from build123d import *

# Parameters (mm, degrees)
F0_W     = 20
F0_H     = 120
F1_DEPTH = 25
F2_R     = 2.5
F3_DEPTH = 20.001


with BuildPart() as f1:
    # F0 (on Front) → F1 (new body, symmetric)
    with BuildSketch(Plane.XZ):
        Rectangle(F0_W, F0_H)
        with BuildLine():
            ThreePointArc((87.128021, -54.795358), (51.166331, -95.96169), (10, -60))
            Line((10, -60), (-10, -60))
            ThreePointArc((-10, -60), (51.166331, -115.96169), (107.128021, -54.795358))
            Line((107.128021, -54.795358), (87.128021, -54.795358))
        make_face()
    extrude(amount=F1_DEPTH, both=True)

    # F2 (on face) → F3 (cut, through all)
    with BuildSketch(Plane.YZ.offset(10)):
        with Locations((0, -21.438537)):
            Circle(F2_R)
        with Locations((0, 38.03635)):
            Circle(F2_R)
    extrude(amount=-F3_DEPTH, mode=Mode.SUBTRACT)


solid = f1.part
Verification items for the finished model (mm, model axes). Coordinates: 2 decimals unless noted, no trailing zeros. Order: outer loops, then holes, each group sorted by start corner. A loop starts at its lowest first (then second) coordinate and runs counter-clockwise, first axis right, second up.
1. Release check for a two-part mould opening along X. For faces 1 (the face through (-10, 0, -1)), 2 (the face through (52.014, -0.35, -95.895)), 3 (the face through (50, 0, -116)), 4 (the face through (97, 0, -54.795)) record: +X half, -X half, draft (parallel to the pull), parting line (faces both ways), or undercut.
Results found:
face 1: -X half
face 2: undercut
face 3: parting line
face 4: draft
2. Go/stop test with flat-tipped pins: pin 1 Ø3 at (x, y) = (84, -17) entering from -Z; pin 2 Ø1 at (x, y) = (38.5, 9.5) entering from +Z; pin 3 Ø6 at (x, y) = (93.5, -0.5) entering from +Z. Record where each tip stops, or that it passes through.
Results found:
pin 1: stops at z = -105.2
pin 2: stops at z = -94.58
pin 3: stops at z = -54.8
3. Sectioned sample at D-D, the plane x = 39.5. Record the cut outline in (y, z).
Results found:
outline: (-25, -115.31) - (25, -115.31) - (25, -94.97) - (-25, -94.97) - close
4. Sectioned sample at B-B, the plane z = 44. Record the cut outline in (x, y).
Results found:
outline: (-10, -25) - (10, -25) - (10, 25) - (-10, 25) - close
5. Scan lines: line 1 (X direction, y = 9, z = 29); line 2 (Y direction, x = 3, z = -23.5); line 3 (Z direction, x = -5, y = 0). Record each from-to range of solid material in increasing order.
Results found:
line 1: x = -10 to 10
line 2: y = -25 to -1.41, 1.41 to 25
line 3: z = -81.22 to -23.94, -18.94 to 35.54, 40.54 to 60
6. Sectioned sample at C-C, the plane y = -19. Record the cut outline in (x, z).
Results found:
outline: (-10, -60) arc R58.62 ccw to (107.13, -54.8) - (87.13, -54.8) arc R38.65 cw to (10, -60) - (10, 60) - (-10, 60) - close
7. Sectioned sample at A-A, the plane y = 0. Record the cut outline in (x, z).
Results found:
outline: (-10, -60) arc R58.62 ccw to (107.13, -54.8) - (87.13, -54.8) arc R38.65 cw to (10, -60) - (10, -23.94) - (-10, -23.94) - close; (-10, -18.94) - (10, -18.94) - (10, 35.54) - (-10, 35.54) - close; (-10, 40.54) - (10, 40.54) - (10, 60) - (-10, 60) - close
